Source: CAD feature listing. Evaluate the final solid. Frame: model axes, mm. A direction names the side the tool comes from. Give positions to 0.01 mm unless a question says otherwise; leave off trailing zeros. Write each loop counter-clockwise with the first axis right and the second up, starting at its lowest first coordinate (ties: lowest second). Pieces come first, ordered by that corner, then holes. Notation, with made-up numbers: (-28, -1) -> (-19, -1) arc R10 cw to (-19, 5) -> close; hole circle Ø5 at (3.25, 46). An arc over 180 degrees is marked (long way). Use one line per item in the form item = value. Start each with the question number.
(1) Cut plane D-D, the plane y = 52. Output: boundary loops of the cut face in (x, z).
(2) Cut plane C-C, the plane x = -37.5. Output: boundary loops of the cut face in (y, z).
(3) Cut plane A-A, the plane y = 48. Output: boundary loops of the cut face in (x, z), and give its area (3 significant figures).
(4) Material intervals for line 1 along X through (y, z) = (53.5, 26.5); line 2 along Y through (x, z) = (-44.5, 28.75); line 3 along Y through (x, z) = (-44, 24), sorted ascending. Write a range as from..to.
(5) Set-up query: faces 1 (the face through (-46, 48, 26)), 2 (the face through (-36, 51, 24)). Return all of +Z, -Z, +X, -X, +Y, -Y with unobstructed straight access to the full face (end or side cutting, diameter ignored); none if empty.
(6) Cut plane B-B, the plane z = 26. Output: boundary loops of the cut face in (x, y).
from build123d import *

# Parameters (mm, degrees)
CYLINDER_R                   = 3.4
CYLINDER_DEPTH               = 10
BOX003_W                     = 22
BOX003_H                     = 10
BOX003_DEPTH                 = 15
FUSION002004_PLACEMENT_ANGLE = 90


with BuildPart() as cylinder:
    # Cylinder → Cylinder (new body)
    with BuildSketch(Plane(origin=(-10, 5, 9), x_dir=(0, 0, -1), z_dir=(1, 0, 0))):
        Circle(CYLINDER_R)
    extrude(amount=CYLINDER_DEPTH)


with BuildPart() as potentiometer:
    # Box003 → Box003 (new body)
    with BuildSketch(Plane.XY):
        with Locations((11, 5)):
            Rectangle(BOX003_W, BOX003_H)
    extrude(amount=BOX003_DEPTH)

    # Fusion002004: union Cylinder
    add(cylinder.part)


with BuildPart() as potentiometer_1:
    # Fusion002004 placement: moved
    add(potentiometer.part.moved(Location((-36, 57, 21))).rotate(Axis((-36, 57, 21), (1, 0, 0)), FUSION002004_PLACEMENT_ANGLE))


solid = potentiometer_1.part
Geometry says:
q1.outline = (-36, 21) -> (-14, 21) -> (-14, 31) -> (-36, 31) -> close
q2.outline = circle Ø6.8 at (48, 26)
q3.outline = (-46, 22.6) -> (-36, 22.6) -> (-36, 21) -> (-14, 21) -> (-14, 31) -> (-36, 31) -> (-36, 29.4) -> (-46, 29.4) -> close
q3.area = 288 mm^2
q4.line_1 = -36..-14
q4.line_2 = 46..50
q4.line_3 = 45.25..50.75
q5.face_1 = +Z, -Z, -X, +Y, -Y
q5.face_2 = -X
q6.outline = (-46, 44.6) -> (-36, 44.6) -> (-36, 42) -> (-14, 42) -> (-14, 57) -> (-36, 57) -> (-36, 51.4) -> (-46, 51.4) -> close
